from build123d import *

# Parameters (mm, degrees)
BOSS_EXTRUDE1_REACH      = 150.085
BOSS_EXTRUDE1_END_RADIUS = 60.96
BOSS_EXTRUDE1_START      = -38.1
SKETCH2_R                = 21.59
SKETCH2_R_2              = 17.145


with BuildPart() as part:
    # Sketch1 → Revolve1 (revolve)
    with BuildSketch(Plane.XY):
        with BuildLine():
            Line((-63.5, 0), (-60.96, 0))
            ThreePointArc((-60.96, 0), (-21.552614691, 57.022858574), (45.72, 40.321249981))
            Line((45.72, 40.321249981), (45.72, 44.067352995))
            ThreePointArc((45.72, 44.067352995), (-23.759524406, 58.887477446), (-63.5, 0))
        make_face()
    revolve(axis=Axis((-63.5, 0, 0), (1, 0, 0)))

    # Boss-Extrude1: up to this sphere (the profile starts inside it)
    boss_extrude1_end = Location((0, 0, 0)) * Sphere(BOSS_EXTRUDE1_END_RADIUS, mode=Mode.PRIVATE)
    # Sketch2 → Boss-Extrude1 (add, up to the surface)
    with BuildSketch(Plane(origin=(0, 0, 0), x_dir=(0, 0, -1), z_dir=(1, 0, 0)).offset(BOSS_EXTRUDE1_START), mode=Mode.PRIVATE) as boss_extrude1_sk1:
        with Locations((0, 10.0076)):
            Circle(SKETCH2_R)
        with Locations((0, 10.0076)):
            Circle(SKETCH2_R_2, mode=Mode.SUBTRACT)
    boss_extrude1_tool1 = extrude(boss_extrude1_sk1.sketch, amount=-BOSS_EXTRUDE1_REACH, mode=Mode.PRIVATE) & boss_extrude1_end
    add(boss_extrude1_tool1.solids().sort_by_distance((-38.1, 10.0076, 20.979343))[0])


solid = part.part
CAD build for the part. Positions are in the model's coordinates, mm. Coordinates: 2 decimals unless noted, no trailing zeros. Loops run counter-clockwise (first coordinate to the right, second up) from the corner with the lowest first, then second, coordinate; pieces in that order, holes last. Notation, with made-up numbers: (64, 50.5) - (113, 50.5) arc R6 cw to (113, 56.5) - close; hole circle Ø2 at (-16, -3). An arc over 180 degrees is marked (long way). Use one line per item in the form item = value. Start each with the question number.
1) Band-saw the part on C-C (y = 16). Give the cut face in (x, z).
2) Band-saw the part on A-A (x = -40). Give the cut face in (y, z) (3 decimals), and give its area (3 significant figures).
3) Flat gauge pins, fed straight in: pin 1 (1 mm diameter, centred on y = -28.5, z = -6, fed in from +X); pin 2 (2 mm diameter, centred on x = 7, y = -3, fed in from -Z); pin 3 (5 mm diameter, centred on x = 9.5, z = 12, fed in from +Y). Where does each tip first touch, or does it go through?
4) Band-saw the part on D-D (z = 0). Give the cut face in (x, y), and give its area (3 significant figures).
5) Band-saw the part on B-B (z = -19). Give the cut face in (x, y).
6) Two-plate mould, pull along Z, no slides. Class faces 1 (the face through (45.72, -19, -36)), 2 (the face through (-38.1, 28, -1)): +Z half, -Z half, draft (parallel to the pull), parting line (faces both ways), or undercut.
7) Drill centre lines: L1, parallel to Y at x = -52, z = 0; L2, parallel to Y at x = -43.25, z = 0; L3, parallel to Y at x = -33, z = -44. Where is each one in solid material? Low to high. Write a range as from..to.
Check values:
q1.outline = (-56.59, -16.06) arc R58.82 cw to (-56.59, 16.06) - (-38.1, 16.06) - (-38.1, 20.74) - (-55.04, 20.74) arc R58.82 cw to (45.72, 37.01) - (45.72, 41.06) arc R61.45 ccw (long way) to (45.72, -41.06) - (45.72, -37.01) arc R58.82 cw to (-55.04, -20.74) - (-38.1, -20.74) - (-38.1, -16.06) - close
q2.outline = circle Ø98.636 at (0, 0); circle Ø43.18 at (10.008, 0); hole circle Ø92.003 at (0, 0); hole circle Ø34.29 at (10.008, 0)
q2.area = 1,530 mm2
q3.pin_1 = -53.28
q3.pin_2 = -63.15
q3.pin_3 = 62.2
q4.outline = (-60.54, -7.14) arc R60.96 cw to (-54.58, 27.15) - (-38.1, 27.15) - (-38.1, 31.6) - (-52.13, 31.6) arc R60.96 cw to (45.72, 40.32) - (45.72, 44.07) arc R63.5 ccw (long way) to (45.72, -44.07) - (45.72, -40.32) arc R60.96 cw to (-59.85, -11.58) - (-38.1, -11.58) - (-38.1, -7.14) - close
q4.area = 924 mm2
q5.outline = (-57.92, -0.25) - (-38.1, -0.25) - (-38.1, 20.26) - (-54.26, 20.26) arc R57.92 cw to (45.72, 35.56) - (45.72, 39.76) arc R60.59 ccw (long way) to (45.72, -39.76) - (45.72, -35.56) arc R57.92 cw to start
q6.face_1 = draft
q6.face_2 = undercut
q7.L1 = -36.45..-31.81, -11.58..-7.14, 27.15..31.6, 31.81..36.45
q7.L2 = -46.49..-42.96, -11.58..-7.14, 27.15..31.6, 42.96..46.49
q7.L3 = -31.74..-26.29, 26.29..31.74
